```python
from build123d import *

# Parameters (mm, degrees)
SKETCH2_W           = 200
SKETCH2_H           = 300
BOSS_EXTRUDE1_DEPTH = 5
SKETCH4_W           = 200
SKETCH4_H           = 300
SKETCH4_W_2         = 190
SKETCH4_H_2         = 290
BOSS_EXTRUDE2_DEPTH = 120
SKETCH5_W           = 190
SKETCH5_H           = 5
BOSS_EXTRUDE3_DEPTH = 150
SKETCH7_R           = 7.5
CUT_EXTRUDE1_DEPTH  = 215
FILLET4_R           = 2.5


with BuildPart() as part:
    # Sketch2 → Boss-Extrude1 (new body)
    with BuildSketch(Plane(origin=(0, 0, 0), x_dir=(1, 0, 0), z_dir=(0, 1, 0))):
        Rectangle(SKETCH2_W, SKETCH2_H)
    extrude(amount=BOSS_EXTRUDE1_DEPTH)

    # Sketch4 → Boss-Extrude2 (add)
    with BuildSketch(Plane(origin=(0, 5, 0), x_dir=(1, 0, 0), z_dir=(0, 1, 0))):
        Rectangle(SKETCH4_W, SKETCH4_H)
        Rectangle(SKETCH4_W_2, SKETCH4_H_2, mode=Mode.SUBTRACT)
    extrude(amount=BOSS_EXTRUDE2_DEPTH)

    # Sketch5 → Boss-Extrude3 (add)
    with BuildSketch(Plane(origin=(0, 0, 145), x_dir=(-1, 0, 0), z_dir=(0, 0, -1))):
        with Locations((0, 122.5)):
            Rectangle(SKETCH5_W, SKETCH5_H)
    extrude(amount=BOSS_EXTRUDE3_DEPTH)

    # Sketch7 → Cut-Extrude1 (cut, symmetric)
    with BuildSketch(Plane(origin=(-95, 0, 0), x_dir=(0, 0, -1), z_dir=(1, 0, 0))):
        with Locations(Location((-80, 20, 0), (0, 0, 180))):
            Circle(SKETCH7_R)
    extrude(amount=CUT_EXTRUDE1_DEPTH, both=True, mode=Mode.SUBTRACT)

    # Fillet4
    fillet4_edges = [part.edges().sort_by_distance(p)[0] for p in [
        (95, 20, 72.5),
        (-95, 20, 72.5),
        (-100, 20, 72.5),
        (100, 20, 72.5),
    ]]
    fillet(fillet4_edges, radius=FILLET4_R - 0.0001)  # a hair under: the kernel refuses the full size


solid = part.part
```
Geometry: final body of the model. Coordinates: model frame, mm. A direction names the side the tool comes from. Coordinates: 2 decimals unless noted, no trailing zeros. Loops run counter-clockwise (first coordinate to the right, second up) from the corner with the lowest first, then second, coordinate; pieces in that order, holes last. Notation, with made-up numbers: (8.5, 29) -> (26.5, 29) arc R21 cw to (26.5, 37) -> close; hole circle Ø8 at (76, 51.25). An arc over 180 degrees is marked (long way). Use a Markdown table: item, result. Add a question column.
(1) Line query: line 1 along Z through (x, y) = (45, 52); line 2 along X through (y, z) = (41.5, -118.5); line 3 along Y through (x, z) = (-86.5, 3.5). Output: solid intervals per line, ascending.
(2) Access query for faces 1 (the flat face through (-1, 64, -145)), 2 (the flat face through (-1, 62, 145)), 3 (the flat face through (100, 62, 2)). Directions: +Z, -Z, +X, -X, +Y, -Y. A direction counts if a zero-diameter tool reaches every point of the face in a straight line with its end or side. Return the directions, or none.
(3) Section query C-C, the plane z = -73. Return loops of the section in (x, y).
(4) Mould query, pull axis Z, two halves, no side actions, for faces 4 (the flat face through (-1, 125, 65)), 5 (the flat face through (-1, 5, -2)), 6 (the flat face through (-1, 62, -150)), 7 (the flat face through (1, 120, 71)). Classes: pulls with the +Z half, pulls with the -Z half, needs draft (parallel to the pull), parting line crosses it, or undercut.
(5) Section query D-D, the plane y = 53. Return loops of the section in (x, z).
(6) Pin query (flat end, axial travel): pin 1 Ø24 at (y, z) = (20, 80) entering from -X; pin 2 Ø1.5 at (x, z) = (53.5, -48) entering from +Y. Return the tip coordinate at first contact, or that it passes through.
Answer:
| question | item | result |
|---|---|---|
| 1 | line 1 | z = -150 to -145, 145 to 150 |
| 1 | line 2 | x = -100 to -95, 95 to 100 |
| 1 | line 3 | y = 0 to 5, 120 to 125 |
| 2 | face 1 | +Y |
| 2 | face 2 | none |
| 2 | face 3 | +Z, -Z, +X, +Y, -Y |
| 3 | outline | (-100, 0) -> (100, 0) -> (100, 125) -> (95, 125) -> (95, 5) -> (-95, 5) -> (-95, 125) -> (-100, 125) -> close |
| 4 | face 4 | needs draft |
| 4 | face 5 | undercut |
| 4 | face 6 | pulls with the -Z half |
| 4 | face 7 | undercut |
| 5 | outline | (-100, -150) -> (100, -150) -> (100, 150) -> (-100, 150) -> close; hole (-95, -145) -> (95, -145) -> (95, 145) -> (-95, 145) -> close |
| 6 | pin 1 | stops at x = -100 |
| 6 | pin 2 | stops at y = 5 |
